Read the model definition and answer for the solid it produces. Units are mm, in the model's axes. A direction names the side the tool comes from. Round coordinates to 2 decimals unless told otherwise and drop trailing zeros. Order: outer loops, then holes, each group sorted by start corner. A loop starts at its lowest first (then second) coordinate and runs counter-clockwise, first axis right, second up. Notation, with made-up numbers: (68.25, 13.25) -> (90.25, 13.25) arc R14 cw to (90.25, 22.25) -> close; hole circle Ø4 at (-33, 10). An arc over 180 degrees is marked (long way). Use a Markdown table: item, result. Add a question column.
1. Section C-C, the plane y = 13.75 is taken. Give the vertices of the cut face in (x, z), then the cut area to 3 significant figures.
2. Section D-D, the plane y = 16.25 is taken. Give the vertices of the cut face in (x, z), then the cut area to 3 significant figures.
3. For faces 1 (the face through (0, 7, -6)), 2 (the face through (-4, 0, 4)), determine the directions among +Z, -Z, +X, -X, +Y, -Y from which every point of the face is accessible in a straight line to the end or side of a thin tool.
4. Section A-A, the plane x = 0 is taken. Give the vertices of the cut face in (y, z).
5. Section B-B, the plane z = 0 is taken. Give the vertices of the cut face in (x, y), then the cut area to 3 significant figures.
6. Given pin 1 (3 mm diameter, centred on x = -4, z = -3, fed in from +Y); pin 2 (3 mm diameter, centred on x = 0, z = 2, fed in from -Y); pin 3 (4 mm diameter, centred on x = -4.5, z = -4, fed in from +Y), each flat-ended and moving along its own axis, determine where each tip first touches the part or whether it passes through.
7. The mould has two halves that part along X. Classify faces 3 (the face through (-2, 13.5, -6)), 4 (the face through (2.681, 14.007, 6.466)), 5 (the face through (-4.88, 3.7, 1.08)): +X half, -X half, draft (parallel to the pull), parting line (faces both ways), or undercut.
8. Consider L1, parallel to X at y = 2.75, z = 0; L2, parallel to X at y = 4.75, z = 4.25; L3, parallel to Z at x = 4.5, y = 5. Determine where each line is inside the solid, lowest interval first. Write a range as [from, to].
```python
from build123d import *

# Parameters (mm, degrees)
DOME2_FACE_RADIUS  = 4.35
DOME2_HEIGHT       = 3
SKETCH6_R          = 5
CUT_EXTRUDE1_DEPTH = 7.5


with BuildPart() as part:
    # Sketch1 → Revolve1 (revolve)
    with BuildSketch(Plane(origin=(0, 0, 0), x_dir=(0, 0, -1), z_dir=(1, 0, 0))):
        Polygon((0, 0), (-6, 0), (-6, 13.5), (-7, 13.5), (-7, 14.5), (-4.75, 16), (-4.35, 15), (0, 15), align=None)
    revolve(axis=Axis((0, 15, 0), (0, -1, 0)))

    # Dome2: a dome of height H over a round flat face of radius A is a cap of a sphere of radius (A * A + H * H) / (2 * H)
    dome2_r = (DOME2_FACE_RADIUS * DOME2_FACE_RADIUS + DOME2_HEIGHT * DOME2_HEIGHT) / (2 * DOME2_HEIGHT)
    dome2_base = Plane((0, 15, 0), z_dir=(0, 1, 0))
    with Locations(dome2_base.offset(DOME2_HEIGHT - dome2_r)):
        dome2_ball = Sphere(dome2_r, mode=Mode.PRIVATE)
    add(split(dome2_ball, bisect_by=dome2_base, keep=Keep.TOP, mode=Mode.PRIVATE))

    # Sketch6 → Cut-Extrude1 (cut)
    with BuildSketch(Plane.XZ):
        with Locations(Location((0, 0, 0), (0, 0, 270))):
            Circle(SKETCH6_R)
    extrude(amount=-CUT_EXTRUDE1_DEPTH, mode=Mode.SUBTRACT)


solid = part.part
```
Verdict:
| question | item | result |
|---|---|---|
| 1 | outline | circle Ø14 at (0, 0) |
| 1 | area | 154 mm2 |
| 2 | outline | circle Ø7.27 at (0, 0) |
| 2 | area | 41.5 mm2 |
| 3 | face 1 | -Y |
| 3 | face 2 | +Z, -Z, +X, -X, -Y |
| 4 | outline | (0, -6) -> (13.5, -6) -> (13.5, -7) -> (14.5, -7) -> (16, -4.75) -> (15, -4.35) arc R4.65 ccw to (15, 4.35) -> (16, 4.75) -> (14.5, 7) -> (13.5, 7) -> (13.5, 6) -> (0, 6) -> (0, 5) -> (7.5, 5) -> (7.5, -5) -> (0, -5) -> close |
| 5 | outline | (-7, 13.5) -> (-6, 13.5) -> (-6, 0) -> (-5, 0) -> (-5, 7.5) -> (5, 7.5) -> (5, 0) -> (6, 0) -> (6, 13.5) -> (7, 13.5) -> (7, 14.5) -> (4.75, 16) -> (4.35, 15) arc R4.65 ccw to (-4.35, 15) -> (-4.75, 16) -> (-7, 14.5) -> close |
| 5 | area | 128 mm2 |
| 6 | pin 1 | stops at y = 16.41 |
| 6 | pin 2 | stops at y = 7.5 |
| 6 | pin 3 | stops at y = 16 |
| 7 | face 3 | draft |
| 7 | face 4 | parting line |
| 7 | face 5 | undercut |
| 8 | L1 | x = [-6, -5], [5, 6] |
| 8 | L2 | x = [-4.24, -2.63], [2.63, 4.24] |
| 8 | L3 | z = [-3.97, -2.18], [2.18, 3.97] |
